For this review, use the dimensioned drawing (mm, ordinates from the lowest corner) and the shaded views. A direction names the side the tool comes from. Give positions to 0.01 mm unless a question says otherwise; leave off trailing zeros. Order: outer loops, then holes, each group sorted by start corner. A loop starts at its lowest first (then second) coordinate and runs counter-clockwise, first axis right, second up.
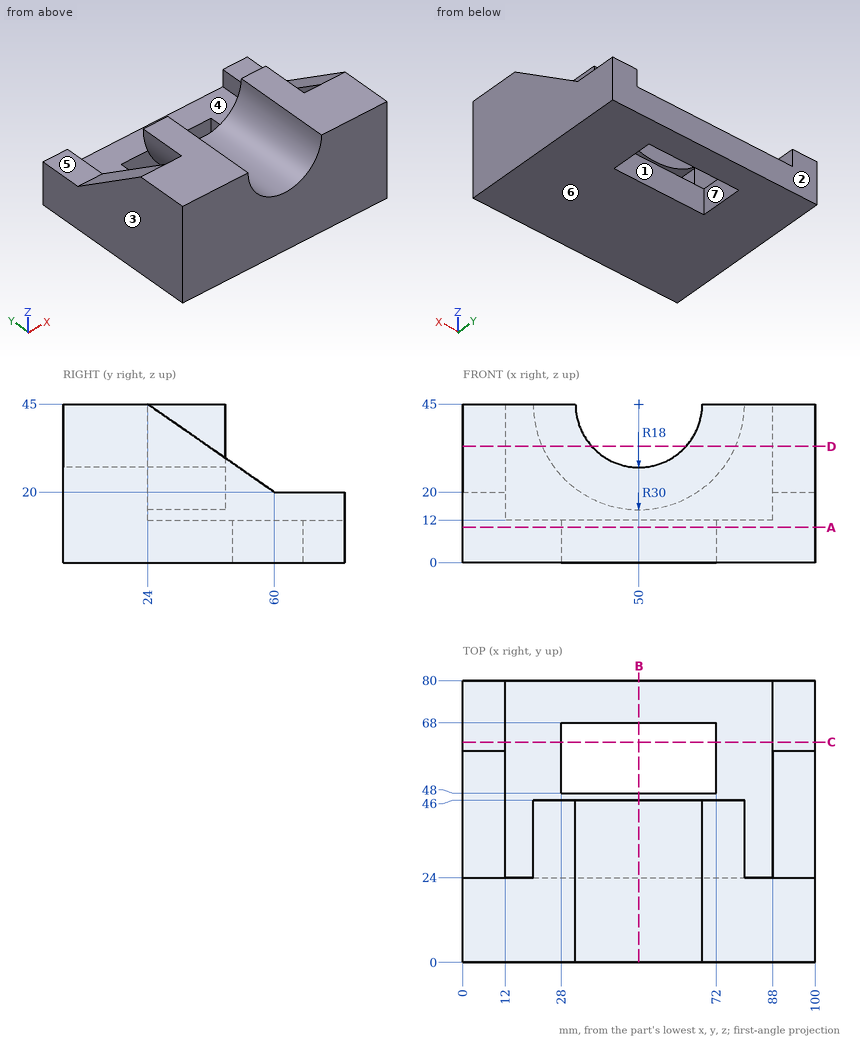
1. Take a section at B-B (x = 50). State the section outline as (y, z) points.
Recorded:
outline: (0, 0) - (48, 0) - (48, 12) - (24, 12) - (24, 15) - (46, 15) - (46, 27) - (0, 27) - close; (68, 0) - (80, 0) - (80, 12) - (68, 12) - close
2. Machinability: for the marked faces 4, 5, 6 and 7, which of the approach directions +Z, -Z, +X, -X, +Y, -Y give a long, thin tool a straight path to every point of the face, cutting with its end or side? Answer none if there is none.
Recorded:
face 4: +Y
face 5: +Z, +X, -X, +Y
face 6: -Z, +X, -X, +Y, -Y
face 7: +Z, -Z
3. Take a section at D-D (z = 33). State the section outline as (x, y) points.
Recorded:
outline: (0, 0) - (36.58, 0) - (36.58, 46) - (22.5, 46) - (22.5, 24) - (12, 24) - (12, 41.28) - (0, 41.28) - close; (63.42, 0) - (100, 0) - (100, 41.28) - (88, 41.28) - (88, 24) - (77.5, 24) - (77.5, 46) - (63.42, 46) - close
4. For pin 1 (2 mm diameter, centred on x = 81, z = 14, fed in from +Y); pin 2 (13 mm diameter, centred on x = 92.5, y = 65.5, fed in from +Z); pin 3 (16.5 mm diameter, centred on x = 44.5, z = 23.5, fed in from +Y); pin 4 (10 mm diameter, centred on y = 52, z = 35.5, fed in from -X), all flat-tipped, find the tip position at first contact; note any pin that passes through.
Recorded:
pin 1: stops at y = 24
pin 2: stops at z = 20.69
pin 3: stops at y = 46
pin 4: passes through
5. Take a section at A-A (z = 10). State the section outline as (x, y) points.
Recorded:
outline: (0, 0) - (100, 0) - (100, 80) - (0, 80) - close; hole (28, 48) - (72, 48) - (72, 68) - (28, 68) - close
6. Draft analysis for pull direction X (two halves, no side actions). For the marked faces 1, 2 and 3, state which applies: pulls with the +X half, pulls with the -X half, needs draft (parallel to the pull), parting line crosses it, or undercut.
Recorded:
face 1: undercut
face 2: needs draft
face 3: pulls with the -X half
7. For line 1 along X through (y, z) = (61, 7); line 2 along Y through (x, z) = (36.5, 11.5); line 3 along X through (y, z) = (76.5, 15), list the stretches that pass through material, from the lowest coordinate up.
Recorded:
line 1: x = 0 to 28, 72 to 100
line 2: y = 0 to 48, 68 to 80
line 3: x = 0 to 12, 88 to 100
8. Take a section at C-C (y = 62.5). State the section outline as (x, z) points, then the cut area to 3 significant figures.
Recorded:
outline: (0, 0) - (28, 0) - (28, 12) - (12, 12) - (12, 20) - (0, 20) - close; (72, 0) - (100, 0) - (100, 20) - (88, 20) - (88, 12) - (72, 12) - close
area: 864 mm2
